```python
from build123d import *

# Parameters (mm, degrees)
BOSS_EXTRUDE1_DEPTH            = 33.31
CUT_EXTRUDE1_DEPTH             = 85.661420376
CUT_EXTRUDE1_DEPTH_BACK        = 85.661420376
SKETCH2_R                      = 5.5
FILLET1_R                      = 10
CUT_EXTRUDE2_REACH             = 86.661
SKETCH3_R                      = 5.5
CUT_EXTRUDE3_DEPTH             = 82.379088837
CUT_EXTRUDE3_DEPTH_BACK        = 82.379088837
SKETCH4_R                      = 1.225
CUT_EXTRUDE4_REACH             = 86.661
SKETCH6_R                      = 1.35
CUT_EXTRUDE4_DIRECTION_2_DEPTH = 85.661420376


with BuildPart() as part:
    # Sketch1 → Boss-Extrude1 (new body)
    with BuildSketch(Plane(origin=(0, 0, 0), x_dir=(1, 0, 0), z_dir=(0, 1, 0))):
        Polygon((0, 57), (0, 0), (53, 0), (53, 5), (5, 5), (5, 52), (53, 52), (53, 57), align=None)
    extrude(amount=BOSS_EXTRUDE1_DEPTH)

    # Sketch2 → Cut-Extrude1 (cut, two sides: drawn at the far end of the back side and taken through both)
    with BuildSketch(Plane.XY.offset(-CUT_EXTRUDE1_DEPTH_BACK)):
        with Locations((37, 16.655)):
            Circle(SKETCH2_R)
    extrude(amount=CUT_EXTRUDE1_DEPTH + CUT_EXTRUDE1_DEPTH_BACK, mode=Mode.SUBTRACT)

    # Fillet1
    fillet1_edges = [part.edges().sort_by_distance(p)[0] for p in [
        (53, 0, -54.5),
        (53, 33.31, -54.5),
        (53, 33.31, -2.5),
        (53, 0, -2.5),
    ]]
    fillet(fillet1_edges, radius=FILLET1_R)

    # Sketch3 → Cut-Extrude2 (cut, up to next)
    with BuildSketch(Plane.ZY, mode=Mode.PRIVATE) as cut_extrude2_sk1:
        with Locations((-28.5, 16.655)):
            Circle(SKETCH3_R)
    cut_extrude2_tool1 = extrude(cut_extrude2_sk1.sketch, amount=-CUT_EXTRUDE2_REACH, mode=Mode.PRIVATE) & part.part
    add(cut_extrude2_tool1.solids().sort_by_distance((0, 16.655, -28.5))[0], mode=Mode.SUBTRACT)

    # Sketch4 → Cut-Extrude3 (cut, two sides: drawn at the far end of the back side and taken through both)
    with BuildSketch(Plane(origin=(0, 0, -5), x_dir=(-1, 0, 0), z_dir=(0, 0, -1)).offset(-CUT_EXTRUDE3_DEPTH_BACK)):
        with Locations((-37.902229443, 27.617936743)):
            Circle(SKETCH4_R)
        with Locations((-29.886005644, 25.04493947)):
            Circle(SKETCH4_R)
        with Locations((-26.037063257, 17.557229443)):
            Circle(SKETCH4_R)
        with Locations((-28.61006053, 9.541005644)):
            Circle(SKETCH4_R)
        with Locations((-36.097770557, 5.692063257)):
            Circle(SKETCH4_R)
        with Locations((-44.113994356, 8.26506053)):
            Circle(SKETCH4_R)
        with Locations((-47.962936743, 15.752770557)):
            Circle(SKETCH4_R)
        with Locations((-45.38993947, 23.768994356)):
            Circle(SKETCH4_R)
    extrude(amount=CUT_EXTRUDE3_DEPTH + CUT_EXTRUDE3_DEPTH_BACK, mode=Mode.SUBTRACT)

    # Sketch6 → Cut-Extrude4 (cut, up to next)
    with BuildSketch(Plane.ZY, mode=Mode.PRIVATE) as cut_extrude4_sk1:
        with Locations(Location((-20.963129564, 8.642785323, 0), (0, 0, 180))):
            Circle(SKETCH6_R)
    cut_extrude4_tool1 = extrude(cut_extrude4_sk1.sketch, amount=-CUT_EXTRUDE4_REACH, mode=Mode.PRIVATE) & part.part
    # Sketch6 → Cut-Extrude4 (cut, up to next)
    with BuildSketch(Plane.ZY, mode=Mode.PRIVATE) as cut_extrude4_sk2:
        with Locations(Location((-28.836119137, 5.660136475, 0), (0, 0, 180))):
            Circle(SKETCH6_R)
    cut_extrude4_tool2 = extrude(cut_extrude4_sk2.sketch, amount=-CUT_EXTRUDE4_REACH, mode=Mode.PRIVATE) & part.part
    # Sketch6 → Cut-Extrude4 (cut, up to next)
    with BuildSketch(Plane.ZY, mode=Mode.PRIVATE) as cut_extrude4_sk3:
        with Locations(Location((-36.512214677, 9.118129564, 0), (0, 0, 180))):
            Circle(SKETCH6_R)
    cut_extrude4_tool3 = extrude(cut_extrude4_sk3.sketch, amount=-CUT_EXTRUDE4_REACH, mode=Mode.PRIVATE) & part.part
    # Sketch6 → Cut-Extrude4 (cut, up to next)
    with BuildSketch(Plane.ZY, mode=Mode.PRIVATE) as cut_extrude4_sk4:
        with Locations(Location((-39.494863525, 16.991119137, 0), (0, 0, 180))):
            Circle(SKETCH6_R)
    cut_extrude4_tool4 = extrude(cut_extrude4_sk4.sketch, amount=-CUT_EXTRUDE4_REACH, mode=Mode.PRIVATE) & part.part
    # Sketch6 → Cut-Extrude4 (cut, up to next)
    with BuildSketch(Plane.ZY, mode=Mode.PRIVATE) as cut_extrude4_sk5:
        with Locations(Location((-36.036870436, 24.667214677, 0), (0, 0, 180))):
            Circle(SKETCH6_R)
    cut_extrude4_tool5 = extrude(cut_extrude4_sk5.sketch, amount=-CUT_EXTRUDE4_REACH, mode=Mode.PRIVATE) & part.part
    # Sketch6 → Cut-Extrude4 (cut, up to next)
    with BuildSketch(Plane.ZY, mode=Mode.PRIVATE) as cut_extrude4_sk6:
        with Locations(Location((-28.163880863, 27.649863525, 0), (0, 0, 180))):
            Circle(SKETCH6_R)
    cut_extrude4_tool6 = extrude(cut_extrude4_sk6.sketch, amount=-CUT_EXTRUDE4_REACH, mode=Mode.PRIVATE) & part.part
    # Sketch6 → Cut-Extrude4 (cut, up to next)
    with BuildSketch(Plane.ZY, mode=Mode.PRIVATE) as cut_extrude4_sk7:
        with Locations(Location((-20.487785323, 24.191870436, 0), (0, 0, 180))):
            Circle(SKETCH6_R)
    cut_extrude4_tool7 = extrude(cut_extrude4_sk7.sketch, amount=-CUT_EXTRUDE4_REACH, mode=Mode.PRIVATE) & part.part
    # Sketch6 → Cut-Extrude4 (cut, up to next)
    with BuildSketch(Plane.ZY, mode=Mode.PRIVATE) as cut_extrude4_sk8:
        with Locations(Location((-17.505136475, 16.318880863, 0), (0, 0, 180))):
            Circle(SKETCH6_R)
    cut_extrude4_tool8 = extrude(cut_extrude4_sk8.sketch, amount=-CUT_EXTRUDE4_REACH, mode=Mode.PRIVATE) & part.part
    add(cut_extrude4_tool1.solids().sort_by_distance((0, 8.642785, -20.96313))[0], mode=Mode.SUBTRACT)
    add(cut_extrude4_tool2.solids().sort_by_distance((0, 5.660136, -28.836119))[0], mode=Mode.SUBTRACT)
    add(cut_extrude4_tool3.solids().sort_by_distance((0, 9.11813, -36.512215))[0], mode=Mode.SUBTRACT)
    add(cut_extrude4_tool4.solids().sort_by_distance((0, 16.991119, -39.494864))[0], mode=Mode.SUBTRACT)
    add(cut_extrude4_tool5.solids().sort_by_distance((0, 24.667215, -36.03687))[0], mode=Mode.SUBTRACT)
    add(cut_extrude4_tool6.solids().sort_by_distance((0, 27.649864, -28.163881))[0], mode=Mode.SUBTRACT)
    add(cut_extrude4_tool7.solids().sort_by_distance((0, 24.19187, -20.487785))[0], mode=Mode.SUBTRACT)
    add(cut_extrude4_tool8.solids().sort_by_distance((0, 16.318881, -17.505136))[0], mode=Mode.SUBTRACT)

    # Sketch6 → Cut-Extrude4 direction 2 (cut)
    with BuildSketch(Plane.ZY):
        with Locations(Location((-20.963129564, 8.642785323, 0), (0, 0, 180))):
            Circle(SKETCH6_R)
        with Locations(Location((-28.836119137, 5.660136475, 0), (0, 0, 180))):
            Circle(SKETCH6_R)
        with Locations(Location((-36.512214677, 9.118129564, 0), (0, 0, 180))):
            Circle(SKETCH6_R)
        with Locations(Location((-39.494863525, 16.991119137, 0), (0, 0, 180))):
            Circle(SKETCH6_R)
        with Locations(Location((-36.036870436, 24.667214677, 0), (0, 0, 180))):
            Circle(SKETCH6_R)
        with Locations(Location((-28.163880863, 27.649863525, 0), (0, 0, 180))):
            Circle(SKETCH6_R)
        with Locations(Location((-20.487785323, 24.191870436, 0), (0, 0, 180))):
            Circle(SKETCH6_R)
        with Locations(Location((-17.505136475, 16.318880863, 0), (0, 0, 180))):
            Circle(SKETCH6_R)
    extrude(amount=CUT_EXTRUDE4_DIRECTION_2_DEPTH, mode=Mode.SUBTRACT)


solid = part.part
```
CAD build for the part. Positions are in the model's coordinates, mm. A direction names the side the tool comes from. Give positions to 0.01 mm unless a question says otherwise; leave off trailing zeros. Loops run counter-clockwise (first coordinate to the right, second up) from the corner with the lowest first, then second, coordinate; pieces in that order, holes last. Notation, with made-up numbers: (2, -9.5) - (58, -9.5) arc R21 ccw to (58, 11.5) - close; hole circle Ø5 at (8.25, 15). An arc over 180 degrees is marked (long way). Put each result on its own line as item: value.
Q1. Slice it at C-C (x = 25.5). Give the cut face in (y, z), plus the area to 3 significant figures.
Filled in:
outline: (0, -57) - (16.46, -57) - (16.46, -52) - (0, -52) - close; (0, -5) - (16.46, -5) - (16.46, 0) - (0, 0) - close; (18.66, -57) - (33.31, -57) - (33.31, -52) - (18.66, -52) - close; (18.66, -5) - (33.31, -5) - (33.31, 0) - (18.66, 0) - close
area: 311 mm²
Q2. Tool access for faces 1 (the face through (29, 16, -5)), 2 (the face through (2.465, 16.897, -33.995)): list every direction of +Z, -Z, +X, -X, +Y, -Y with a clear straight run to the whole face (end or side of a thin tool).
Filled in:
face 1: +X, +Y, -Y
face 2: +X, -X
Q3. Slice it at B-B (z = -17). Give the cut face in (x, y), plus the area to 3 significant figures.
Filled in:
outline: (0, 0) - (5, 0) - (5, 15.07) - (0, 15.07) - close; (0, 17.57) - (5, 17.57) - (5, 33.31) - (0, 33.31) - close
area: 154 mm²
Q4. Probe line 1 along Z through (x, y) = (7, 19); line 2 along Z through (x, y) = (4.5, 8.5); line 3 along X through (y, z) = (5, -20). List the from-to ranges inside material, lowest first.
Filled in:
line 1: z = -57 to -52, -5 to 0
line 2: z = -57 to -37.71, -35.31 to -22.31, -19.62 to 0
line 3: x = 0 to 5
Q5. Slice it at D-D (z = -28.5). Give the cut face in (x, y) (3 decimals), plus the area to 3 significant figures.
Filled in:
outline: (0, 0) - (5, 0) - (5, 4.353) - (0, 4.353) - close; (0, 6.968) - (5, 6.968) - (5, 11.155) - (0, 11.155) - close; (0, 22.155) - (5, 22.155) - (5, 26.342) - (0, 26.342) - close; (0, 28.957) - (5, 28.957) - (5, 33.31) - (0, 33.31) - close
area: 85.4 mm²
Q6. Mould opens along X. For faces 3 (the face through (2.46, 7.73, -19.97)), 4 (the face through (53, 17, -2)), 5 (the face through (29.834, 9.595, -54.465)) say: pulls with the +X half, pulls with the -X half, needs draft (parallel to the pull), parting line crosses it, or undercut.
Filled in:
face 3: needs draft
face 4: pulls with the +X half
face 5: undercut
Q7. Flat gauge pins, fed straight in: pin 1 (2 mm diameter, centred on x = 37.9, y = 27.62, fed in from -Z); pin 2 (4.5 mm diameter, centred on y = 24.19, z = -20.49, fed in from +X). Where does each tip first touch, or does it go through?
Filled in:
pin 1: passes through
pin 2: stops at x = 5
Q8. Slice it at A-A (x = 8). Give the cut face in (y, z).
Filled in:
outline: (0, -57) - (33.31, -57) - (33.31, -52) - (0, -52) - close; (0, -5) - (33.31, -5) - (33.31, 0) - (0, 0) - close
